Verification items for the finished model (mm, model axes). Face numbers are marked on the shaded views. A direction names the side the tool comes from. Coordinates: 2 decimals unless noted, no trailing zeros. Loops run counter-clockwise (first coordinate to the right, second up) from the corner with the lowest first, then second, coordinate; pieces in that order, holes last. Notation, with made-up numbers: (43, 54.5) -> (79, 54.5) arc R22 ccw to (79, 89.5) -> close; hole circle Ø2 at (17.25, 15). An arc over 180 degrees is marked (long way). Write item = value, one per line.
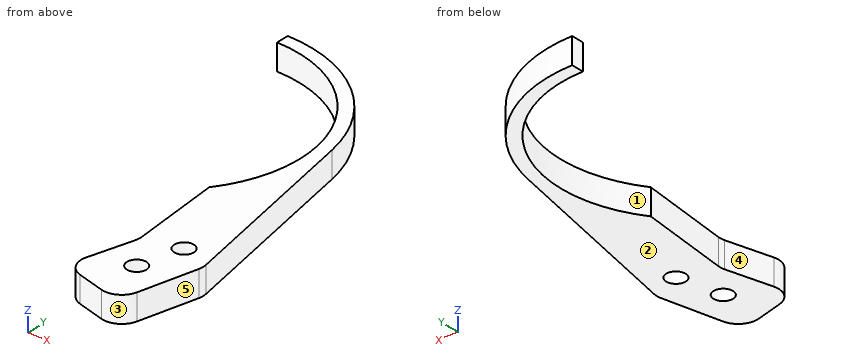
```python
from build123d import *

# Parameters (mm, degrees)
SKETCH_1_R      = 1.5
EXTRUDE_1_DEPTH = 4
FILLET_1_R      = 3


with BuildPart() as part:
    # 草图1 → 凸台-拉伸1 (new body)
    with BuildSketch(Plane.XY):
        with BuildLine():
            Line((-10.940603829, 79.049047398), (-10.940603829, 81.049047398))
            ThreePointArc((-10.940603829, 81.049047398), (3.025840458, 76.047236536), (10.641601769, 63.316177759))
            Line((10.641601769, 63.316177759), (16.862252241, 31.85349767))
            Line((16.862252241, 31.85349767), (13.93581935, 19.153521371))
            Line((13.93581935, 19.153521371), (3.838956556, 21.858772904))
            Line((3.838956556, 21.858772904), (6.612464071, 32.210388823))
            Line((6.612464071, 32.210388823), (5.095703598, 47.097610493))
            ThreePointArc((5.095703598, 47.097610493), (6.934361039, 68.020425829), (-10.940603829, 79.049047398))
        make_face()
        with Locations((10.520263625, 27.067195715)):
            Circle(SKETCH_1_R, mode=Mode.SUBTRACT)
        with Locations((12.212445248, 33.85958273)):
            Circle(SKETCH_1_R, mode=Mode.SUBTRACT)
    extrude(amount=EXTRUDE_1_DEPTH)

    # 圆角1
    fillet_1_edges = [part.edges().sort_by_distance(p)[0] for p in [
        (16.862252241, 31.85349767, 2),
        (13.93581935, 19.153521371, 2),
        (3.838956556, 21.858772904, 2),
        (6.612464071, 32.210388823, 2),
    ]]
    fillet(fillet_1_edges, radius=FILLET_1_R)


solid = part.part
```
1) Tool access check on the marked faces 4 and 5. Record the directions out of +Z, -Z, +X, -X, +Y, -Y that give a thin tool (end or side, any length) a straight path to the whole face; none if there is none.
Ans:
face_4 = +Z, -Z, -X
face_5 = +Z, -Z, +X, -Y
2) Release check for a two-part mould opening along Y. For the marked faces 1, 2 and 3 record: pulls with the +Y half, pulls with the -Y half, needs draft (parallel to the pull), parting line crosses it, or undercut.
Ans:
face_1 = undercut
face_2 = needs draft
face_3 = pulls with the -Y half
3) Sectioned sample at B-B, the plane x = -0.5. Record the cut outline in (y, z).
Ans:
outline = (76.11, 0) -> (78.41, 0) -> (78.41, 4) -> (76.11, 4) -> close
4) Material ranges on line 1 (Y direction, x = 7.25, z = 2.6); line 2 (X direction, y = 34, z = 1.55); line 3 (X direction, y = 72.5, z = 3.75), recorded low to high.
Ans:
line_1 = 20.94 to 50.74, 67.36 to 71.42
line_2 = 6.43 to 10.72, 13.71 to 16.44
line_3 = 3.86 to 6.47
5) Sectioned sample at C-C, the plane y = 69.5. Record the cut outline in (x, z), plus the area to 3 significant figures.
Ans:
outline = (6.11, 0) -> (8.42, 0) -> (8.42, 4) -> (6.11, 4) -> close
area = 9.23 mm2
6) Depth check by flat-ended pin: pin 1 Ø2.5 at (x, y) = (10.52, 27.07) entering from +Z; pin 2 Ø1.5 at (x, z) = (-5.5, 1.5) entering from -Y; pin 3 Ø1 at (y, z) = (30, 3) entering from +X; pin 4 Ø6 at (x, y) = (13, 62) entering from -Z. Enter the tip coordinate at first touch or a pass-through.
Ans:
pin_1 = through
pin_2 = 78.07
pin_3 = 16.55
pin_4 = 0
7) Sectioned sample at A-A, the plane z = 0.85. Record the cut outline in (x, y), plus the area to 3 significant figures.
Ans:
outline = (-10.94, 79.05) arc R20 cw to (5.1, 47.1) -> (6.56, 32.76) arc R3 cw to (6.47, 31.68) -> (4.62, 24.76) arc R3 ccw to (6.74, 21.08) -> (10.93, 19.96) arc R3 ccw to (14.63, 22.18) -> (16.72, 31.23) arc R3 ccw to (16.74, 32.48) -> (10.64, 63.32) arc R22 ccw to (-10.94, 81.05) -> close; hole circle Ø3 at (10.52, 27.07); hole circle Ø3 at (12.21, 33.86)
area = 371 mm2
